For this review, take the finished solid that the model builds, in its own axes (mm). A direction names the side the tool comes from. Coordinates: 2 decimals unless noted, no trailing zeros. Order: outer loops, then holes, each group sorted by start corner. A loop starts at its lowest first (then second) coordinate and runs counter-clockwise, first axis right, second up. Notation, with made-up numbers: M -5.75,44.5 L 19.25,44.5 A22 ccw 19.25,72.5 Z; hole C 37.5,42 d2. An arc over 180 degrees is marked long. Use one line per item in the form item = value. Start each with the question number.
```python
from build123d import *

# Parameters (mm, degrees)
F0_W     = 91
F0_H     = 138
F1_DEPTH = 25
F2_R     = 10
F3_R     = 6.25
F4_DEPTH = 103.001


with BuildPart() as f1:
    # F0 (on Front) → F1 (new body, symmetric)
    with BuildSketch(Plane.XZ):
        Polygon((45.5, 0), (-45.5, 0), (-45.696307, 250), (-51.5, 250), (-51.5, -350), (-45.5, -350), (-45.5, -150), (45.5, -150), (45.5, -350), (51.5, -350), (51.5, 250), (45.5, 250), align=None)
        with Locations((0, -75)):
            Rectangle(F0_W, F0_H, mode=Mode.SUBTRACT)
    extrude(amount=F1_DEPTH, both=True)

    # F2
    f2_edges = [f1.edges().sort_by_distance(p)[0] for p in [
        (48.5, -25, 250),
        (48.5, 25, 250),
        (-48.598153, -25, 250),
        (-48.598153, 25, 250),
        (48.5, -25, -350),
        (-48.5, -25, -350),
        (48.5, 25, -350),
        (-48.5, 25, -350),
    ]]
    fillet(f2_edges, radius=F2_R)

    # F3 (on face) → F4 (cut, through all)
    with BuildSketch(Plane.YZ.offset(51.5)):
        with Locations((0, 200)):
            Circle(F3_R)
        with Locations((0, 100)):
            Circle(F3_R)
    extrude(amount=-F4_DEPTH, mode=Mode.SUBTRACT)


solid = f1.part
```
1. Consider section A-A, the plane z = -60. Write out the cut boundary in (x, y), plus the area to 3 significant figures.
2. To check wall thickness, follow line 1 (Z direction, x = 47, y = 0); line 2 (X direction, y = 18, z = -253.5); line 3 (Z direction, x = 12, y = -8.5). State the ranges of each line that lie inside material, in increasing order.
3. Tool access review of faces 4 (the flat face through (-1, 0, -6)), 5 (the flat face through (1, 0, 0)), 6 (the cylindrical face through (-48.63, 21.99, 247.15)), 7 (the flat face through (45.5, 0, -249)), 8 (the cylindrical face through (-48.63, -21.99, 247.15)): name each direction out of +Z, -Z, +X, -X, +Y, -Y from which nothing blocks a thin tool from reaching the whole face with its end or side.
4. Consider section B-B, the plane x = -15.5. Write out the cut boundary in (y, z), plus the area to 3 significant figures.
5. Consider section C-C, the plane y = 0. Give the number of separate pieces and of enclosed holes in the cut face, plus the area to 3 significant figures.
6. Consider section D-D, the plane z = 200. Write out the cut boundary in (x, y).
7. The part is to be moulded in two halves that separate along Z. For faces 1 (the cylindrical face through (48.46, 21.99, 247.15)), 2 (the cylindrical face through (48.54, -21.99, -347.15)), 3 (the flat face through (-1, 0, -144)), say which applies: pulls with the +Z half, pulls with the -Z half, needs draft (parallel to the pull), parting line crosses it, or undercut.
8. For pin 1 Ø15 at (x, y) = (4, 11.5) entering from -Z; pin 2 Ø6 at (x, y) = (-39, 13) entering from +Z; pin 3 Ø7.5 at (y, z) = (0, 200) entering from +X, all flat-tipped, find the tip position at first contact; note any pin that passes through.
Answers follow:
q1.outline = M -51.5,-25 L -45.5,-25 L -45.5,25 L -51.5,25 Z; M 45.5,-25 L 51.5,-25 L 51.5,25 L 45.5,25 Z
q1.area = 600 mm²
q2.line_1 = -350 to 93.75, 106.25 to 193.75, 206.25 to 250
q2.line_2 = -51.5 to -45.5, 45.5 to 51.5
q2.line_3 = -150 to -144, -6 to 0
q3.face_4 = +Y, -Y
q3.face_5 = +Z, +Y, -Y
q3.face_6 = +Z, +X, -X, +Y
q3.face_7 = -Z, +Y, -Y
q3.face_8 = +Z, +X, -X, -Y
q4.outline = M -25,-150 L 25,-150 L 25,-144 L -25,-144 Z; M -25,-6 L 25,-6 L 25,0 L -25,0 Z
q4.area = 600 mm²
q5.separate_pieces = 5
q5.enclosed_holes = 1
q5.area = 7,970 mm²
q6.outline = M -51.5,-25 L -45.66,-25 L -45.66,-6.25 L -51.5,-6.25 Z; M -51.5,6.25 L -45.66,6.25 L -45.66,25 L -51.5,25 Z; M 45.5,-25 L 51.5,-25 L 51.5,-6.25 L 45.5,-6.25 Z; M 45.5,6.25 L 51.5,6.25 L 51.5,25 L 45.5,25 Z
q7.face_1 = pulls with the +Z half
q7.face_2 = pulls with the -Z half
q7.face_3 = undercut
q8.pin_1 = -150
q8.pin_2 = 0
q8.pin_3 = through
